```python
from build123d import *

# Parameters (mm, degrees)
SKETCH1_W           = 40
SKETCH1_H           = 60
SKETCH1_R           = 14
BOSS_EXTRUDE1_DEPTH = 27
SKETCH2_W           = 40
SKETCH2_H           = 60
SKETCH2_R           = 13
BOSS_EXTRUDE2_DEPTH = 3


with BuildPart() as part:
    # Sketch1 → Boss-Extrude1 (new body)
    with BuildSketch(Plane.XY):
        Rectangle(SKETCH1_W, SKETCH1_H)
        Circle(SKETCH1_R, mode=Mode.SUBTRACT)
    extrude(amount=BOSS_EXTRUDE1_DEPTH)

    # Sketch2 → Boss-Extrude2 (add)
    with BuildSketch(Plane(origin=(0, 0, 0), x_dir=(-1, 0, 0), z_dir=(0, 0, -1))):
        Rectangle(SKETCH2_W, SKETCH2_H)
        Circle(SKETCH2_R, mode=Mode.SUBTRACT)
    extrude(amount=BOSS_EXTRUDE2_DEPTH)


solid = part.part
```
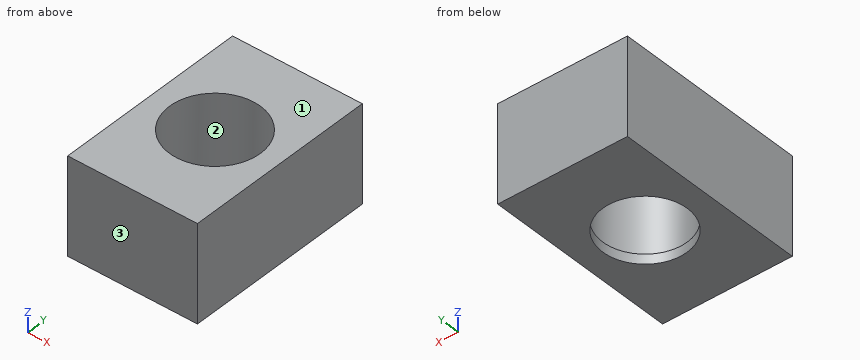
Build history of the part. All positions in model axes, mm. Face numbers are marked on the shaded views. Give positions to 0.01 mm unless a question says otherwise; leave off trailing zeros. Loops run counter-clockwise (first coordinate to the right, second up) from the corner with the lowest first, then second, coordinate; pieces in that order, holes last. Notation, with made-up numbers: (3, -27.75) -> (51, -27.75) arc R33 cw to (51, 3.25) -> close; hole circle Ø5 at (40, 74). An arc over 180 degrees is marked (long way). One line per question, with ' | ' between items. Start each with the question number.
1) Cut at C-C (z = 20.75). Give the cut face in (x, y), plus the area to 3 significant figures.
2) Cut at B-B (x = 0). Give the cut face in (y, z), plus the area to 3 significant figures.
3) Probe L1, parallel to Y at x = 0, z = 11.25; L2, parallel to Y at x = -5.5, z = 25.75; L3, parallel to Z at x = 12, y = 6.5. List the from-to ranges inside material, lowest first.
4) Two-plate mould, pull along Y, no slides. Class the marked faces 1, 2 and 3: released by +Y, released by -Y, zero draft, split by the parting line, or undercut.
5) Cut at A-A (y = 0). Give the cut face in (x, z).
Return value:
1) outline: (-20, -30) -> (20, -30) -> (20, 30) -> (-20, 30) -> close; hole circle Ø28 at (0, 0) | area: 1,780 mm^2
2) outline: (-30, -3) -> (-13, -3) -> (-13, 0) -> (-14, 0) -> (-14, 27) -> (-30, 27) -> close; (13, -3) -> (30, -3) -> (30, 27) -> (14, 27) -> (14, 0) -> (13, 0) -> close | area: 966 mm^2
3) L1: -30 to -14, 14 to 30 | L2: -30 to -12.87, 12.87 to 30 | L3: -3 to 0
4) face 1: zero draft | face 2: undercut | face 3: released by -Y
5) outline: (-20, -3) -> (-13, -3) -> (-13, 0) -> (-14, 0) -> (-14, 27) -> (-20, 27) -> close; (13, -3) -> (20, -3) -> (20, 27) -> (14, 27) -> (14, 0) -> (13, 0) -> close
